Design review of the part built by this model. Coordinates are the model's own, in mm. Face numbers are marked on the shaded views. Give positions to 0.01 mm unless a question says otherwise; leave off trailing zeros. Loops run counter-clockwise (first coordinate to the right, second up) from the corner with the lowest first, then second, coordinate; pieces in that order, holes last. Notation, with made-up numbers: (14.5, 89) -> (45.5, 89) arc R27 ccw to (45.5, 128) -> close; hole circle Ø4 at (-28, 49.5). An arc over 180 degrees is marked (long way). Answer in a Markdown table with one row per item. Add a question column.
(1) Consider section B-B on z = 0. Write out the cut boundary in (x, y) (3 decimals).
(2) Draft analysis for pull direction X (two halves, no side actions). For the marked faces 1, 2 and 3, state which applies: +X half, -X half, draft (parallel to the pull), parting line (faces both ways), or undercut.
(3) Consider section A-A on x = 0. Write out the cut boundary in (y, z) (3 decimals), then the cut area to 3 significant figures.
(4) For line 1 (Z direction, x = 0, y = 7.75) (3 decimals); line 2 (Z direction, x = 2.5, y = 1), list the stretches that pass through material, from the lowest coordinate up.
(5) For pin 1 (4 mm diameter, centred on x = -9.5, y = 7, fed in from -Z); pin 2 (6 mm diameter, centred on x = -12, y = 10, fed in from +Z); pin 3 (2 mm diameter, centred on x = -2, y = 7, fed in from -Z), all flat-tipped, find the tip position at first contact; note any pin that passes through.
(6) Consider section C-C on y = 7. Write out the cut boundary in (x, z) (3 decimals), then the cut area to 3 significant figures.
from build123d import *

# Parameters (mm, degrees)
SKETCH1_R           = 18.595
BOSS_EXTRUDE1_DEPTH = 11
SKETCH2_R           = 4.125
CUT_EXTRUDE1_DEPTH  = 12
CHAMFER1_SIZE       = 1


with BuildPart() as part:
    # Sketch1 → Boss-Extrude1 (new body)
    with BuildSketch(Plane(origin=(0, 0, 0), x_dir=(1, 0, 0), z_dir=(0, 1, 0))):
        Circle(SKETCH1_R)
    extrude(amount=BOSS_EXTRUDE1_DEPTH)

    # Sketch2 → Cut-Extrude1 (cut, through all)
    with BuildSketch(Plane(origin=(0, 11, 0), x_dir=(1, 0, 0), z_dir=(0, 1, 0))):
        Circle(SKETCH2_R)
    extrude(amount=-CUT_EXTRUDE1_DEPTH, mode=Mode.SUBTRACT)

    # Chamfer1
    chamfer1_edges = [part.edges().sort_by_distance(p)[0] for p in [
        (-18.595, 0, 0),
        (-18.595, 11, 0),
    ]]
    chamfer(chamfer1_edges, length=CHAMFER1_SIZE)


solid = part.part
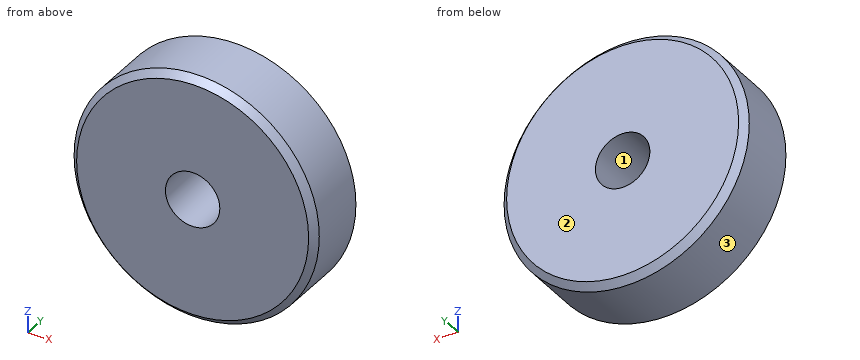
Values follow:
| question | item | result |
|---|---|---|
| 1 | outline | (-18.595, 1) -> (-17.595, 0) -> (-4.125, 0) -> (-4.125, 11) -> (-17.595, 11) -> (-18.595, 10) -> close; (4.125, 0) -> (17.595, 0) -> (18.595, 1) -> (18.595, 10) -> (17.595, 11) -> (4.125, 11) -> close |
| 2 | face 1 | undercut |
| 2 | face 2 | draft |
| 2 | face 3 | parting line |
| 3 | outline | (0, -17.595) -> (1, -18.595) -> (10, -18.595) -> (11, -17.595) -> (11, -4.125) -> (0, -4.125) -> close; (0, 4.125) -> (11, 4.125) -> (11, 17.595) -> (10, 18.595) -> (1, 18.595) -> (0, 17.595) -> close |
| 3 | area | 316 mm2 |
| 4 | line 1 | -18.595 to -4.125, 4.125 to 18.595 |
| 4 | line 2 | -18.43 to -3.28, 3.28 to 18.43 |
| 5 | pin 1 | z = -17.02 |
| 5 | pin 2 | z = 16.27 |
| 5 | pin 3 | z = -18.57 |
| 6 | outline | circle Ø37.19 at (0, 0); hole circle Ø8.25 at (0, 0) |
| 6 | area | 1,030 mm2 |
